Design review of the part built by this model. Coordinates are the model's own, in mm. A direction names the side the tool comes from. Give positions to 0.01 mm unless a question says otherwise; leave off trailing zeros. Loops run counter-clockwise (first coordinate to the right, second up) from the corner with the lowest first, then second, coordinate; pieces in that order, holes last. Notation, with made-up numbers: (-27.5, 15) - (-9.5, 15) arc R10 ccw to (-9.5, 21) - close; hole circle Ø8 at (-25.75, -21). An arc over 180 degrees is marked (long way). One line per item, written item: value. Start each with the question number.
```python
from build123d import *

# Parameters (mm, degrees)
PAD_DEPTH    = 30
THICKNESS_T  = -3
SKETCH001_R  = 4
PAD001_DEPTH = 27


with BuildPart() as part:
    # Sketch → Pad (new body)
    with BuildSketch(Plane.XY):
        with BuildLine():
            ThreePointArc((-50, 25), (-57.071068, 22.071068), (-60, 15))
            Line((-60, -15), (-60, 15))
            ThreePointArc((-60, -15), (-57.071068, -22.071068), (-50, -25))
            Line((50, -25), (-50, -25))
            ThreePointArc((50, -25), (57.071068, -22.071068), (60, -15))
            Line((60, 15), (60, -15))
            ThreePointArc((60, 15), (57.071068, 22.071068), (50, 25))
            Line((-50, 25), (50, 25))
        make_face()
    extrude(amount=PAD_DEPTH)

    # Thickness
    thickness_openings = [part.faces().sort_by_distance(p)[0] for p in [
        (0, 0, 30),
    ]]
    offset(amount=THICKNESS_T, openings=thickness_openings)

    # Sketch001 (on Face19 of Thickness) → Pad001 (join)
    with BuildSketch(Plane.XY.offset(3)):
        with Locations((-50, 15)):
            Circle(SKETCH001_R)
        with Locations((-50, -15)):
            Circle(SKETCH001_R)
        with Locations((50, 15)):
            Circle(SKETCH001_R)
        with Locations((50, -15)):
            Circle(SKETCH001_R)
    extrude(amount=PAD001_DEPTH)


solid = part.part
```
(1) Take a section at A-A on z = 13.75. State the section outline as (x, y) points.
(2) Take a section at B-B on x = 28.5. State the section outline as (y, z) points, and give its area (3 significant figures).
(3) Draft analysis for pull direction Y (two halves, no side actions). For faces 1 (the cylindrical face through (-57.15, -21.99, 14.79)), 2 (the cylindrical face through (-54.9, 20, 16.3)), 3 (the flat face through (-1, 25, 15)), state which applies: pulls with the +Y half, pulls with the -Y half, needs draft (parallel to the pull), parting line crosses it, or undercut.
(4) To check wall thickness, follow L1, parallel to Y at x = 35.5, z = 19.5; L2, parallel to X at y = 16, z = 11.5; L3, parallel to X at y = -9, z = 23. State the ranges of each line that lie inside material, in increasing order. Write a range as from..to.
(5) For pin 1 Ø13 at (x, y) = (-25, -7.5) entering from +Z, flat-tipped, find the tip position at first contact; note if it passes through.
(6) Machinability: for faces 4 (the flat face through (-1, 0, 3)), 5 (the flat face through (1, -25, 15)), which of the approach directions +Z, -Z, +X, -X, +Y, -Y give a long, thin tool a straight path to every point of the face, cutting with its end or side? Answer none if there is none.
(7) Take a section at C-C on y = 3.5. State the section outline as (x, z) points.
Here are the results:
1. outline: (-60, -15) arc R10 ccw to (-50, -25) - (50, -25) arc R10 ccw to (60, -15) - (60, 15) arc R10 ccw to (50, 25) - (-50, 25) arc R10 ccw to (-60, 15) - close; circle Ø8 at (-50, -15); circle Ø8 at (-50, 15); circle Ø8 at (50, -15); circle Ø8 at (50, 15); hole (-57, -15) arc R7 ccw to (-50, -22) - (50, -22) arc R7 ccw to (57, -15) - (57, 15) arc R7 ccw to (50, 22) - (-50, 22) arc R7 ccw to (-57, 15) - close
2. outline: (-25, 0) - (25, 0) - (25, 30) - (22, 30) - (22, 3) - (-22, 3) - (-22, 30) - (-25, 30) - close
2. area: 312 mm²
3. face 1: pulls with the -Y half
3. face 2: undercut
3. face 3: pulls with the +Y half
4. L1: -25..-22, 22..25
4. L2: -59.95..-56.93, -53.87..-46.13, 46.13..53.87, 56.93..59.95
4. L3: -60..-57, 57..60
5. pin 1: z = 3
6. face 4: +Z
6. face 5: +Z, -Z, +X, -X, -Y
7. outline: (-60, 0) - (60, 0) - (60, 30) - (57, 30) - (57, 3) - (-57, 3) - (-57, 30) - (-60, 30) - close
